Answer from the drawing. Dimensions are ordinates in mm from the lowest x, y and z of the part. Round coordinates to 2 decimals unless told otherwise and drop trailing zeros. Loops run counter-clockwise (first coordinate to the right, second up) from the corner with the lowest first, then second, coordinate; pieces in that order, holes last. Notation, with made-up numbers: M 33,-27 L 56,-27 A28 cw 56,7 Z; hole C -39.5,26 d2. An arc over 180 degrees is marked long. One line per item, written item: value.
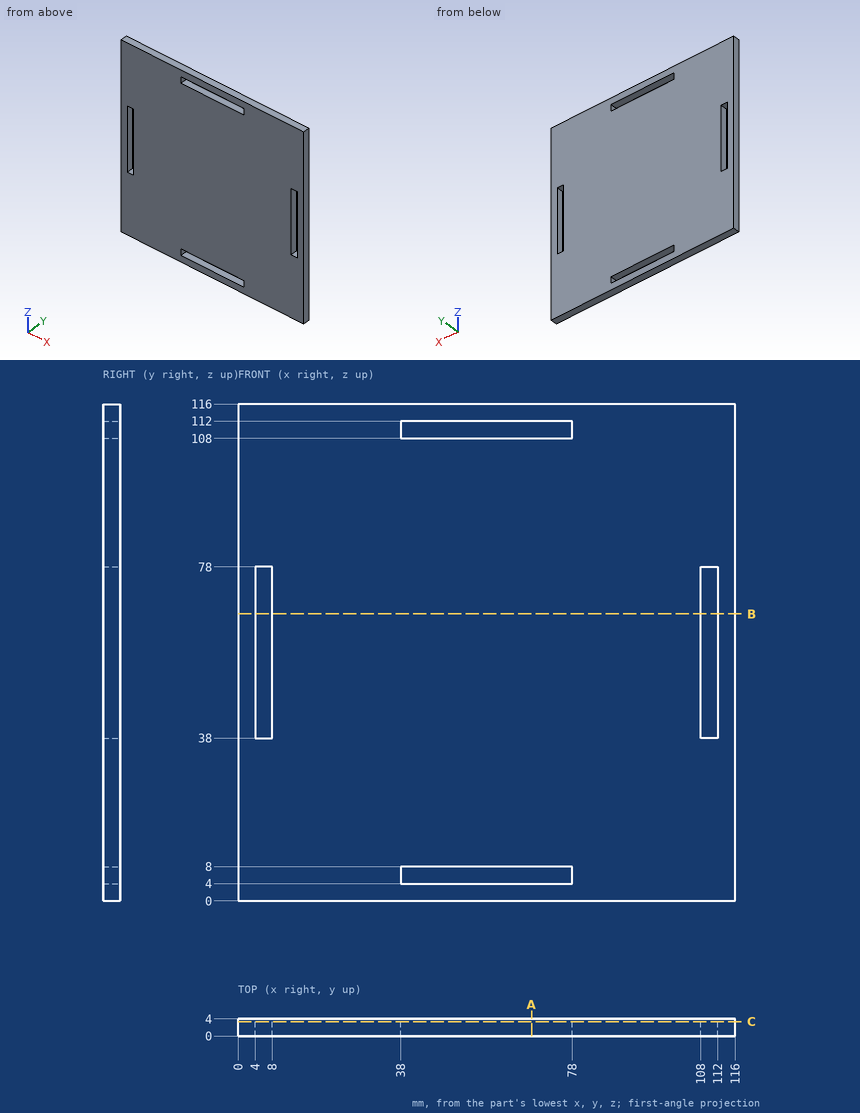
1) Find section B-B (z = 67). Give the vertices of the cut face in (x, y), then the cut area to 3 significant figures.
Check values:
outline: M 0,0 L 4,0 L 4,4 L 0,4 Z; M 8,0 L 108,0 L 108,4 L 8,4 Z; M 112,0 L 116,0 L 116,4 L 112,4 Z
area: 432 mm2
2) Find section A-A (x = 68.5). Give the vertices of the cut face in (y, z).
Check values:
outline: M 0,0 L 4,0 L 4,4 L 0,4 Z; M 0,8 L 4,8 L 4,108 L 0,108 Z; M 0,112 L 4,112 L 4,116 L 0,116 Z
3) Find the intervals of material crossed by probe 1 along X at (y, z) = (0.2, 40); probe 2 along Z at (x, y) = (110, 0.45), in increasing order. Write a range as from..to.
Check values:
probe 1: 0..4, 8..108, 112..116
probe 2: 0..38, 78..116
4) Find section C-C (y = 3.35). Give the vertices of the cut face in (x, z).
Check values:
outline: M 0,0 L 116,0 L 116,116 L 0,116 Z; hole M 4,38 L 8,38 L 8,78 L 4,78 Z; hole M 38,4 L 78,4 L 78,8 L 38,8 Z; hole M 38,108 L 78,108 L 78,112 L 38,112 Z; hole M 108,38 L 112,38 L 112,78 L 108,78 Z
